Source: CAD feature listing. Evaluate the final solid. Frame: model axes, mm. A direction names the side the tool comes from. Round coordinates to 2 decimals unless told otherwise and drop trailing zeros. Loops run counter-clockwise (first coordinate to the right, second up) from the corner with the lowest first, then second, coordinate; pieces in that order, holes last. Notation, with made-up numbers: M -17,-20.75 L 29,-20.75 A16 cw 29,-9.75 Z; hole C 21.25,38.25 d7. An arc over 180 degrees is marked long. One line per item, written item: value.
from build123d import *

# Parameters (mm, degrees)
FILLET1_R   = 0.3556
HEX_2_DEPTH = 3.048


with BuildPart() as part:
    # BodySke → Base-Revolve (revolve)
    with BuildSketch(Plane.XY):
        Polygon((0, 0), (0, 4.1275), (0.635, 4.7625), (6.35, 4.7625), (6.35, 3.175), (37.34435, 3.175), (38.1, 2.41935), (38.1, 0), align=None)
    revolve(axis=Axis((-31.75, 0, 0), (1, 0, 0)))

    # Fillet1
    fillet1_edges = [part.edges().sort_by_distance(p)[0] for p in [
        (6.35, -3.175, 0),
    ]]
    fillet(fillet1_edges, radius=FILLET1_R)

    # Sketch2 → Hex-PreBroach (revolve, cut)
    with BuildSketch(Plane.XY):
        Polygon((0, 2.38125), (3.048, 2.38125), (4.422815329, 0), (0, 0), align=None)
    revolve(axis=Axis((0, 0, 0), (1, 0, 0)), mode=Mode.SUBTRACT)

    # Sketch3 → Hex 2 (cut)
    with BuildSketch(Plane(origin=(0, 0, 0), x_dir=(0, 0.5, 0.866025404), z_dir=(-1, 0, 0))):
        Polygon((1.374815329, 2.38125), (-1.374815329, 2.38125), (-2.749630657, 0), (-1.374815329, -2.38125), (1.374815329, -2.38125), (2.749630657, 0), align=None)
    extrude(amount=-HEX_2_DEPTH, mode=Mode.SUBTRACT)


solid = part.part
1. Ray query, line 1 (X direction, y = -1.5, z = -3.25); line 2 (X direction, y = -0.75, z = -2.25); line 3 (Y direction, x = 15.5, z = 1.5). Return the intervals inside material, ascending. Write a range as [from, to].
Report:
line 1: x = [0, 6.35]
line 2: x = [3.05, 38.1]
line 3: y = [-2.8, 2.8]
2. Section query A-A (x = 33.5). Return the cut outline in (y, z) (3 decimals), and give its area (3 significant figures).
Report:
outline: C 0,0 d6.35
area: 31.7 mm2
3. Pin query (flat end, axial travel): pin 1 (0.6 mm diameter, centred on y = -1, z = 2, fed in from -X); pin 2 (3 mm diameter, centred on x = 31, z = -2, fed in from -Y); pin 3 (4 mm diameter, centred on x = 4, z = 3, fed in from -Y). Return the tip coordinate at first contact, or that it passes through.
Report:
pin 1: stops at x = 3.05
pin 2: stops at y = -3.14
pin 3: stops at y = -4.66
4. Pull-direction query (Y, two-part tool) for faces 4 (the face through (1.503, -2.072, 1.174)), 5 (the face through (0, -2, -2)), 6 (the face through (3.53, -3.78, -2.9)); classes: released by +Y, released by -Y, zero draft, split by the parting line, or undercut.
Report:
face 4: undercut
face 5: zero draft
face 6: split by the parting line
5. Reachability of faces 1 (the face through (1.5, 2.05, 1.21)), 2 (the face through (6.35, -4, 0)), 3 (the face through (38.1, 0, 0)) from +Z, -Z, +X, -X, +Y, -Y: full face, straight path, thin tool, end or side. Return the list, or none.
Report:
face 1: -X
face 2: +X
face 3: +Z, -Z, +X, +Y, -Y
